Read the model definition and answer for the solid it produces. Units are mm, in the model's axes. Face numbers are marked on the shaded views. Give positions to 0.01 mm unless a question says otherwise; leave off trailing zeros. Write each loop counter-clockwise with the first axis right and the second up, starting at its lowest first coordinate (ties: lowest second). Pieces come first, ordered by that corner, then holes. Notation, with made-up numbers: M -36.75,-4.75 L 17.25,-4.75 A12 cw 17.25,6.25 Z; hole C 56,43.5 d6. An arc over 180 degrees is marked long. Write each question's results on one line, items separated by ' | '. Start each with the question number.
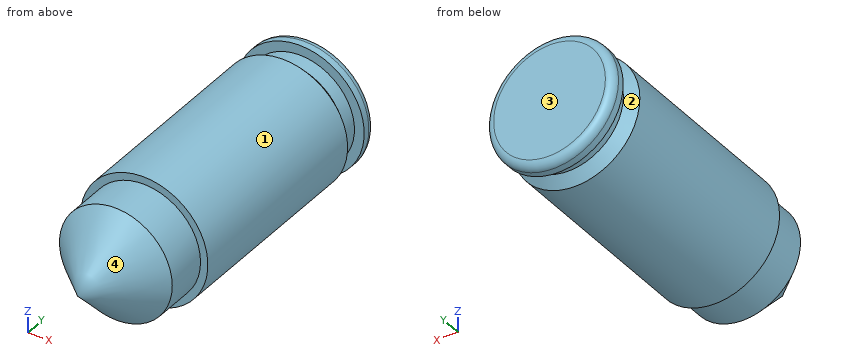
```python
from build123d import *

# Parameters (mm, degrees)
F0_R     = 5.75
F1_DEPTH = 10
F2_SIZE  = 5.75
F3_R     = 6.5
F4_DEPTH = 22
F5_SIZE  = 1
F6_R     = 5.5
F7_DEPTH = 1.5
F8_R     = 6.5
F9_DEPTH = 1.5
F10_R    = 0.8


with BuildPart() as f1:
    # F0 (on Front) → F1 (new body)
    with BuildSketch(Plane.XZ):
        Circle(F0_R)
    extrude(amount=F1_DEPTH)

    # F2
    f2_edges = [f1.edges().sort_by_distance(p)[0] for p in [
        (-5.75, -10, 0),
    ]]
    chamfer(f2_edges, length=F2_SIZE)

    # F3 (on face) → F4 (join)
    with BuildSketch(Plane(origin=(0, 0, 0), x_dir=(-1, 0, 0), z_dir=(0, 1, 0))):
        Circle(F3_R)
    extrude(amount=F4_DEPTH)

    # F5
    f5_edges = [f1.edges().sort_by_distance(p)[0] for p in [
        (6.5, 22, 0),
    ]]
    chamfer(f5_edges, length=F5_SIZE)

    # F6 (on face) → F7 (join)
    with BuildSketch(Plane(origin=(0, 22, 0), x_dir=(-1, 0, 0), z_dir=(0, 1, 0))):
        Circle(F6_R)
    extrude(amount=F7_DEPTH)

    # F8 (on face) → F9 (join)
    with BuildSketch(Plane(origin=(0, 23.5, 0), x_dir=(-1, 0, 0), z_dir=(0, 1, 0))):
        Circle(F8_R)
    extrude(amount=F9_DEPTH)

    # F10
    f10_edges = [f1.edges().sort_by_distance(p)[0] for p in [
        (6.5, 25, 0),
    ]]
    fillet(f10_edges, radius=F10_R)


solid = f1.part
```
Item 1: Given P1, Ø2, axis at x = 5, y = 4, coming from the -Z side; P2, Ø6, axis at x = -4, y = 19, coming from the -Z side; P3, Ø3, axis at x = 5, y = -2, coming from the +Z side, each flat-ended and moving along its own axis, determine where each tip first touches the part or whether it passes through.
Item 2: Determine the mould class of the marked faces 1, 2, 3 and 4 for opening direction Y: +Y half, -Y half, draft (parallel to the pull), parting line (faces both ways), or undercut.
Item 3: Straight lines are drawn through the part: line 1 (Y direction, x = 3.25, z = 2.75); line 2 (Y direction, x = -3.5, z = 4.75); line 3 (Y direction, x = 4, z = 4). For each, find the intervals that lie inside material, in ascending order.
Item 4: Section A-A, the plane y = 11.5 is taken. Determine the outline of the cut face in (x, z).
Worked out:
1) P1: stops at z = -5.12 | P2: stops at z = -6.42 | P3: stops at z = 4.56
2) face 1: draft | face 2: undercut | face 3: +Y half | face 4: -Y half
3) line 1: y = -5.74 to 25 | line 2: y = 0 to 21.6, 23.5 to 24.97 | line 3: y = -4.34 to 21.84, 23.5 to 25
4) outline: C 0,0 d13
